Read the model definition and answer for the solid it produces. Units are mm, in the model's axes. A direction names the side the tool comes from. Round coordinates to 2 decimals unless told otherwise and drop trailing zeros. Loops run counter-clockwise (first coordinate to the right, second up) from the corner with the lowest first, then second, coordinate; pieces in that order, holes last. Notation, with made-up numbers: M -32.5,47.5 L -23.5,47.5 A34 cw -23.5,77.5 Z; hole C 5.25,84.25 d7. An arc over 180 degrees is marked long. Write each question's results on one line, items separated by ' | '.
```python
from build123d import *

# Parameters (mm, degrees)
F0_R     = 9.525
F1_DEPTH = 12.7
F2_R     = 6.35
F3_DEPTH = 12.7
F5_DEPTH = 6.35
F6_W     = 17.704927
F6_H     = 25.4
F7_DEPTH = 12.7
F9_DEPTH = 38.1


with BuildPart() as f1:
    # F0 (on Front) → F1 (new body, symmetric)
    with BuildSketch(Plane.XZ):
        Circle(F0_R)
    extrude(amount=F1_DEPTH, both=True)

    # F2 (on Front) → F3 (cut, symmetric)
    with BuildSketch(Plane.XZ):
        Circle(F2_R)
    extrude(amount=F3_DEPTH, both=True, mode=Mode.SUBTRACT)

    # F4 (on Front) → F5 (join, symmetric)
    with BuildSketch(Plane.XZ):
        with BuildLine():
            ThreePointArc((0, -9.525), (-9.525, 0), (0, 9.525))
            Line((0, 9.525), (-19.180335, 9.525))
            Line((-19.180335, 9.525), (-19.180335, -9.525))
            Line((-19.180335, -9.525), (0, -9.525))
        make_face()
    extrude(amount=F5_DEPTH, both=True)

    # F6 (on Front) → F7 (join, symmetric)
    with BuildSketch(Plane.XZ):
        with Locations((-28.032798, 3.175)):
            Rectangle(F6_W, F6_H)
    extrude(amount=F7_DEPTH, both=True)

    # F8 (on Right) → F9 (cut)
    with BuildSketch(Plane.YZ):
        Polygon((12.7, 9.525), (12.7, 15.875), (6.35, 15.875), align=None)
        Polygon((-6.35, 15.875), (-12.7, 15.875), (-12.7, 9.525), align=None)
    extrude(amount=-F9_DEPTH, mode=Mode.SUBTRACT)


solid = f1.part
```
1. Given P1, Ø3, axis at x = 4.5, z = -1, coming from the +Y side; P2, Ø10, axis at y = -2, z = 6.5, coming from the +X side; P3, Ø3, axis at x = -7.5, z = 9.5, coming from the -Y side; P4, Ø1.5, axis at y = -9.5, z = 7, coming from the +X side, each flat-ended and moving along its own axis, determine where each tip first touches the part or whether it passes through.
Completed:
P1: passes through | P2: stops at x = 9.41 | P3: stops at y = -6.35 | P4: stops at x = 7.19
2. Determine the mould class of faces 3 (the face through (-36.885, 0, 3)), 4 (the face through (-9, 0, 9.525)), 5 (the face through (-19.18, 0, 11)) for opening direction X: released by +X, released by -X, zero draft, split by the parting line, or undercut.
Completed:
face 3: released by -X | face 4: zero draft | face 5: undercut
3. Which of the six approach directions +Z, -Z, +X, -X, +Y, -Y give full straight-line access (tool end or side, diameter ignored) to faces 1 (the face through (-27.909, -9.569, 12.656)), 2 (the face through (9.085, -0.178, 2.861))?
Completed:
face 1: +Z, +X, -X, -Y | face 2: none
4. Find section D-D, the plane y = 4.5. Give the vertices of the cut face in (x, z) (3 decimals), then the cut area to 3 significant figures.
Completed:
outline: M -36.885,-9.525 L 0,-9.525 A9.525 ccw 0,9.525 L -19.18,9.525 L -19.18,15.875 L -36.885,15.875 Z; hole C 0,0 d12.7 | area: 831 mm2
5. Find section B-B, the plane z = 0. Give the vertices of the cut face in (x, y) (3 decimals), then the cut area to 3 significant figures.
Completed:
outline: M -36.885,-12.7 L -19.18,-12.7 L -19.18,-6.35 L -9.525,-6.35 L -9.525,-12.7 L -6.35,-12.7 L -6.35,12.7 L -9.525,12.7 L -9.525,6.35 L -19.18,6.35 L -19.18,12.7 L -36.885,12.7 Z; M 6.35,-12.7 L 9.525,-12.7 L 9.525,12.7 L 6.35,12.7 Z | area: 734 mm2
6. Find section A-A, the plane y = -8.75. Give the vertices of the cut face in (x, z) (3 decimals), then the cut area to 3 significant figures.
Completed:
outline: M -36.885,-9.525 L -19.18,-9.525 L -19.18,13.475 L -36.885,13.475 Z; C 0,0 d19.05; hole C 0,0 d12.7 | area: 566 mm2
7. Find section C-C, the plane x = -5. Give the vertices of the cut face in (y, z) (3 decimals).
Completed:
outline: M -12.7,-8.107 L -6.35,-8.107 L -6.35,-9.525 L 6.35,-9.525 L 6.35,-8.107 L 12.7,-8.107 L 12.7,-3.914 L -12.7,-3.914 Z; M -12.7,3.914 L 12.7,3.914 L 12.7,8.107 L 6.35,8.107 L 6.35,9.525 L -6.35,9.525 L -6.35,8.107 L -12.7,8.107 Z
8. Find the intervals of material crossed by L1, parallel to X at y = -3.5, z = 11; L2, parallel to Z at x = 3, y = 0; L3, parallel to X at y = 1.5, z = 0.5, in increasing order.
Completed:
L1: x = -36.89 to -19.18 | L2: z = -9.04 to -5.6, 5.6 to 9.04 | L3: x = -36.89 to -6.33, 6.33 to 9.51
